Autodesk Inventor part; units mm, degrees
ref_plane "Work Plane2" through (0, 0, -15) normal (0, 0, 1) x (1, 0, 0)
ref_plane "YZ Plane" through (0, 0, 0) normal (1, 0, 0) x (0, 1, 0)
ref_plane "XZ Plane" through (0, 0, 0) normal (0, 1, 0) x (-1, 0, 0)
sketch "Unten" plane through (0, 0, 0) normal (0, 0, 1) x (1, 0, 0)
  line L0 (20.5633, 45) -> (20.5633, 5)
  line L1 (60.5633, 5) -> (60.5633, 45)
  line L2 (60.5633, 45) -> (20.5633, 45)
  line L3 (20.5633, 5) -> (60.5633, 5)
  line L4 (105, 50) -> (0, 50)
  line L5 (105, 0) -> (0, 0)
  line L6 (0, 40.5) -> (16, 40.5)
  line L7 (16, 37.5) -> (16, 12.5)
  line L8 (16, 9.5) -> (0, 9.5)
  line L9 (0, 9.5) -> (0, 40.5)
  line L10 (0, 50) -> (0, 0)
  line L11 (105, 50) -> (105, 0)
  circle A0 centre (23.5633, 8) radius 1
  circle A1 centre (57.5633, 42) radius 1
  line L12 (58.5633, 37.1716) -> (58.5633, 8.5)
  line L13 (57.0633, 7) -> (28.3918, 7)
  line L14 (22.5633, 12.8284) -> (22.5633, 41.5)
  line L15 (24.0633, 43) -> (52.7349, 43)
  line L16 (20.0633, 45.5) -> (61.0633, 45.5)
  line L17 (61.0633, 4.5) -> (20.0633, 4.5)
  arc A2 (57.0633, 7) -> (58.5633, 8.5) centre (57.0633, 8.5) ccw
  arc A3 (24.0633, 43) -> (22.5633, 41.5) centre (24.0633, 41.5) ccw
  line L18 (23.1491, 11.4142) -> (26.9776, 7.5858)
  line L19 (54.1491, 42.4142) -> (57.9776, 38.5858)
  arc A4 (16, 37.5) -> (16, 40.5) centre (16, 39) ccw
  arc A5 (16, 9.5) -> (16, 12.5) centre (16, 11) ccw
  line L20 (20.0633, 45.5) -> (20.0633, 4.5)
  line L21 (61.0633, 4.5) -> (61.0633, 45.5)
  line L22 (0, 25) -> (105, 25) construction
  arc A6 (22.5633, 12.8284) -> (23.1491, 11.4142) centre (24.5633, 12.8284) ccw
  arc A7 (26.9776, 7.5858) -> (28.3918, 7) centre (28.3918, 9) ccw
  arc A8 (58.5633, 37.1716) -> (57.9776, 38.5858) centre (56.5633, 37.1716) ccw
  arc A9 (54.1491, 42.4142) -> (52.7349, 43) centre (52.7349, 41) ccw
  line L23 (50, 0) -> (50, 50) construction
  line L24 (48, 39) -> (48, 40.8)
  line L25 (48, 40.8) -> (44.6, 40.8)
  line L26 (44.6, 40.8) -> (44.6, 39)
  line L27 (44.6, 39) -> (48, 39)
  line L28 (36.2594, 22.5) -> (31.2594, 22.5)
  line L29 (31.2594, 22.5) -> (31.2594, 11.5)
  line L30 (31.2594, 11.5) -> (36.2594, 11.5)
  line L31 (36.2594, 11.5) -> (36.2594, 22.5)
  line L32 (43.6, 9.7) -> (43.6, 13.1)
  line L33 (43.6, 13.1) -> (45.4, 13.1)
  line L34 (45.4, 13.1) -> (45.4, 9.7)
  line L35 (45.4, 9.7) -> (43.6, 9.7)
  point P0 (0, 0)
  point P1 (7.5, 14.5)
  point P2 (7.5, 35.5)
  point P3 (58.5633, 38)
  point P4 (27.5633, 7)
  point P5 (53.5633, 43)
  point P6 (22.5633, 12)
  point P7 (65.5633, 25)
  point P8 (44.7594, 25)
  dimension "d0" = 40
  dimension "d1" = 40
  dimension "d185" = 105
  dimension "d196" = 21
  dimension "d217" = 31
  dimension "d267" = 14.5
  dimension "d268" = 14.5
  dimension "d269" = 50
  dimension "d308" = 9.5
  dimension "d329" = 3
  dimension "d341" = 3
  dimension "d342" = 3
  dimension "d343" = 2
  dimension "d344" = 2
  dimension "d390" = 3
  dimension "d391" = 3
  dimension "d419" = 2
  dimension "d420" = 2
  dimension "d421" = 2
  dimension "d423" = 1.5
  dimension "d424" = 1.5
  dimension "d427" = 0.5
  dimension "d428" = 0.5
  dimension "d431" = 3.5
  dimension "d432" = 3.5
  dimension "d450" = 3.5
  dimension "d451" = 3.5
  dimension "d463" = 3
  dimension "d464" = 1.5
  dimension "d465" = 3
  dimension "d466" = 1.5
  dimension "d482" = 2
  dimension "d515" = 5
  dimension "d516" = 11
  dimension "d517" = 3.4
  dimension "d518" = 1.8
  dimension "d519" = 3.4
  dimension "d520" = 1.8
  dimension "d521" = 7.5
  dimension "d522" = 16
extrude "Extrusion40" add sketch "Unten" against normal blind 15 contours L11 L5 L10 L8 A5 L7 A4 L6 L4 | L16 L21 L17 L20
extrude "Extrusion46" add sketch "Unten" against normal blind 6 contours L2 L1 L3 L0
extrude "Extrusion48" cut sketch "Unten" against normal blind 4.4 contours L2 L1 L3 L0 | L12 A2 L13 A7 L18 A6 L14 A3 L15 A9 L19 A8 | L16 L21 L17 L20 | L27 L26 L25 L24 | L31 L30 L29 L28 | L32 L33 L34 L35
extrude "Extrusion41" add sketch "Unten" against normal blind 6 contours L6 A4 L7 A5 L8 L9
hole "Hole14" at (7.5, 14.5, 0) at (7.5, 35.5, 0) direction (0, 0, -1) diameter 4 end through all
chamfer "Chamfer8" distance 2 angle 45 2 edges at (7.5, 37.5, 0) (7.5, 16.5, 0)
sketch "Side" plane through (0, 0, 0) normal (0, -1, 0) x (1, 0, 0)
  line L0 (105, 0) -> (25, 0)
  line L1 (25, -3.6) -> (105, -3.6)
  line L2 (105, -3.6) -> (105, 0)
  line L3 (25, -3.6) -> (25, 0)
  point P0 (0, 0)
  dimension "d412" = 3.6
  dimension "d443" = 80
  dimension "d479" = 80
fillet "Fillet4" radius 10 1 edges at (105, 25, 0)
ref_plane "Work Plane2" through (0, 0, -15) normal (0, 0, 1) x (1, 0, 0)
sketch "Sketch9" plane through (0, 0, -15) normal (0, 0, 1) x (1, 0, 0)
  line L0 (20.0633, 4.5) -> (20.0633, 45.5)
  line L1 (20.0633, 45.5) -> (101.0633, 45.5)
  line L2 (101.0633, 45.5) -> (101.0633, 4.5)
  line L3 (101.0633, 4.5) -> (20.0633, 4.5)
  line L4 (20.0633, 4.5) -> (20.0633, 45.5)
  point P0 (0, 0)
  dimension "d526" = 41
  dimension "d527" = 81
extrude "Extrusion49" cut sketch "Sketch9" along normal blind 3
properties part number "TNS_V3.1_Greiferbacke" material "PVC, Unplasticized"
Geometry check sheet. Reference: the model listing, model coordinates, mm. A direction names the side the tool comes from. Round coordinates to 2 decimals unless told otherwise and drop trailing zeros. Order: outer loops, then holes, each group sorted by start corner. A loop starts at its lowest first (then second) coordinate and runs counter-clockwise, first axis right, second up. Notation, with made-up numbers: M 67,2.5 L 79,2.5 A4 ccw 79,8.5 Z; hole C 48,-19.5 d11. An arc over 180 degrees is marked long. Answer in a Markdown table with one row per item.
(1) Sectioned sample at A-A, the plane x = 46. Record the cut outline in (y, z), and give its area (3 significant figures).
Responses:
| item | result |
|---|---|
| outline | M 0,-15 L 4.5,-15 L 4.5,-12 L 5,-12 L 5,-6 L 7,-6 L 7,-4.4 L 4.5,-4.4 L 4.5,0 L 0,0 Z; M 43,-6 L 45,-6 L 45,-12 L 45.5,-12 L 45.5,-15 L 50,-15 L 50,0 L 45.5,0 L 45.5,-4.4 L 43,-4.4 Z |
| area | 149 mm² |
(2) Sectioned sample at B-B, the plane x = 7.5. Record the cut outline in (y, z), and give its area (3 significant figures).
Responses:
| item | result |
|---|---|
| outline | M 0,-15 L 9.5,-15 L 9.5,-6 L 12.5,-6 L 12.5,-2 L 10.5,0 L 0,0 Z; M 16.5,-6 L 33.5,-6 L 33.5,-2 L 31.5,0 L 18.5,0 L 16.5,-2 Z; M 37.5,-6 L 40.5,-6 L 40.5,-15 L 50,-15 L 50,0 L 39.5,0 L 37.5,-2 Z |
| area | 415 mm² |
(3) Draft check along Y on faces 1 (the face through (53, 0, -7)), 2 (the face through (6.686, 33.537, -1.875)), 3 (the face through (102.15, 24.65, -3.01)), 4 (the face through (17.5, 39, -10.4)). Enter one of: released by +Y, released by -Y, zero draft, split by the parting line, or undercut.
Responses:
| item | result |
|---|---|
| face 1 | released by -Y |
| face 2 | undercut |
| face 3 | zero draft |
| face 4 | undercut |
(4) Sectioned sample at D-D, the plane y = 35.5. State how many separate pieces and enclosed holes the cut face has, and give its area (3 significant figures).
Responses:
| item | result |
|---|---|
| separate pieces | 3 |
| enclosed holes | 0 |
| area | 661 mm² |
(5) Go/stop test with flat-tipped pins: P1, Ø10, axis at x = 16.5, y = 37.5, coming from the +Z side; P2, Ø3, axis at y = 34.5, z = -8, coming from the +X side; P3, Ø6, axis at x = 29.5, y = 41.5, coming from the -Z side; P4, Ø3, axis at y = 30, z = -3, coming from the +X side. Record where each tip stops, or that it passes through.
Responses:
| item | result |
|---|---|
| P1 | stops at z = 0 |
| P2 | stops at x = 104.99 |
| P3 | stops at z = -6 |
| P4 | stops at x = 103.35 |
(6) Sectioned sample at C-C, the plane y = 28. Record the cut outline in (x, z), and give its area (3 significant figures).
Responses:
| item | result |
|---|---|
| outline | M 0,-6 L 16,-6 L 16,-15 L 20.06,-15 L 20.06,-12 L 20.56,-12 L 20.56,-6 L 22.56,-6 L 22.56,-4.4 L 20.06,-4.4 L 20.06,0 L 0,0 Z; M 58.56,-6 L 60.56,-6 L 60.56,-12 L 101.06,-12 L 101.06,-15 L 105,-15 L 105,-10 A10 ccw 95,0 L 61.06,0 L 61.06,-4.4 L 58.56,-4.4 Z |
| area | 689 mm² |
(7) Scan lines: probe 1 along Y at (x, z) = (7.5, -3.55); probe 2 along X at (y, z) = (28, -13.5); probe 3 along Y at (x, z) = (28, -8.75). Record each from-to range of solid material in increasing order. Write a range as from..to.
Responses:
| item | result |
|---|---|
| probe 1 | y = 0..12.5, 16.5..33.5, 37.5..50 |
| probe 2 | x = 16..20.06, 101.06..105 |
| probe 3 | y = 0..5, 45..50 |
(8) Tool access check on faces 5 (the face through (8, 9.5, -10)), 6 (the face through (40.5, 43.3, -4.4)), 7 (the face through (56.037, 40.527, -5.189)), 8 (the face through (60, 45.5, -14)). Record the directions out of +Z, -Z, +X, -X, +Y, -Y that give a thin tool (end or side, any length) a straight path to the whole face; none if there is none.
Responses:
| item | result |
|---|---|
| face 5 | -Z, -X |
| face 6 | +Z |
| face 7 | +Z, -Z |
| face 8 | -Z |
